Part model, mm, in its own coordinate system. A direction names the side the tool comes from. Coordinates: 2 decimals unless noted, no trailing zeros. Write each loop counter-clockwise with the first axis right and the second up, starting at its lowest first coordinate (ties: lowest second). Pieces come first, ordered by that corner, then holes. Notation, with made-up numbers: (14.25, 15) -> (73.25, 15) arc R18 ccw to (73.25, 25) -> close; hole circle Ø10 at (-8, 88). An arc over 180 degrees is marked (long way). Write item = value, one per line.
from build123d import *

# Parameters (mm, degrees)
SKETCH2_W           = 40
SKETCH2_H           = 30
BOSS_EXTRUDE1_DEPTH = 40
SKETCH3_W           = 10
SKETCH3_H           = 30
CUT_EXTRUDE1_DEPTH  = 40
CUT_EXTRUDE2_REACH  = 55.852
SKETCH5_R           = 2
FILLET2_R           = 1


with BuildPart() as part:
    # Sketch2 → Boss-Extrude1 (new body)
    with BuildSketch(Plane(origin=(0, 0, 0), x_dir=(1, 0, 0), z_dir=(0, 1, 0))):
        Rectangle(SKETCH2_W, SKETCH2_H)
    extrude(amount=BOSS_EXTRUDE1_DEPTH)

    # Sketch3 → Cut-Extrude1 (cut)
    with BuildSketch(Plane(origin=(20, 0, 0), x_dir=(0, 0, -1), z_dir=(1, 0, 0))):
        with Locations((5, 20)):
            Rectangle(SKETCH3_W, SKETCH3_H)
    extrude(amount=-CUT_EXTRUDE1_DEPTH, mode=Mode.SUBTRACT)

    # Sketch5 → Cut-Extrude2 (cut, up to next)
    with BuildSketch(Plane.XY.offset(15), mode=Mode.PRIVATE) as cut_extrude2_sk1:
        with Locations((12.5, 7.8)):
            Circle(SKETCH5_R)
    cut_extrude2_tool1 = extrude(cut_extrude2_sk1.sketch, amount=-CUT_EXTRUDE2_REACH, mode=Mode.PRIVATE) & part.part
    # Sketch5 → Cut-Extrude2 (cut, up to next)
    with BuildSketch(Plane.XY.offset(15), mode=Mode.PRIVATE) as cut_extrude2_sk2:
        with Locations((12.5, 32.8)):
            Circle(SKETCH5_R)
    cut_extrude2_tool2 = extrude(cut_extrude2_sk2.sketch, amount=-CUT_EXTRUDE2_REACH, mode=Mode.PRIVATE) & part.part
    # Sketch5 → Cut-Extrude2 (cut, up to next)
    with BuildSketch(Plane.XY.offset(15), mode=Mode.PRIVATE) as cut_extrude2_sk3:
        with Locations((-12.5, 32.8)):
            Circle(SKETCH5_R)
    cut_extrude2_tool3 = extrude(cut_extrude2_sk3.sketch, amount=-CUT_EXTRUDE2_REACH, mode=Mode.PRIVATE) & part.part
    # Sketch5 → Cut-Extrude2 (cut, up to next)
    with BuildSketch(Plane.XY.offset(15), mode=Mode.PRIVATE) as cut_extrude2_sk4:
        with Locations((-12.5, 7.8)):
            Circle(SKETCH5_R)
    cut_extrude2_tool4 = extrude(cut_extrude2_sk4.sketch, amount=-CUT_EXTRUDE2_REACH, mode=Mode.PRIVATE) & part.part
    add(cut_extrude2_tool1.solids().sort_by_distance((12.5, 7.8, 15))[0], mode=Mode.SUBTRACT)
    add(cut_extrude2_tool2.solids().sort_by_distance((12.5, 32.8, 15))[0], mode=Mode.SUBTRACT)
    add(cut_extrude2_tool3.solids().sort_by_distance((-12.5, 32.8, 15))[0], mode=Mode.SUBTRACT)
    add(cut_extrude2_tool4.solids().sort_by_distance((-12.5, 7.8, 15))[0], mode=Mode.SUBTRACT)

    # Fillet2
    fillet2_edges = [part.edges().sort_by_distance(p)[0] for p in [
        (20, 40, 0),
        (0, 40, -15),
        (-20, 40, 0),
        (0, 0, -15),
        (20, 0, 0),
        (0, 0, 15),
        (-20, 0, 0),
        (-20, 20, -15),
        (20, 20, -15),
        (20, 20, 15),
        (-20, 20, 15),
        (0, 40, 15),
    ]]
    fillet(fillet2_edges, radius=FILLET2_R)


solid = part.part
Q1. Pin check, flat tips, straight feed: pin 1 (3 mm diameter, centred on y = 7, z = -8, fed in from -X); pin 2 (2.5 mm diameter, centred on x = -12.5, y = 32.8, fed in from +Z). Stop position of each tip, or through.
Model answer:
pin_1 = through
pin_2 = -10
Q2. Mould opens along X. For faces 4 (the face through (12.24, 34.783, 7.605)), 5 (the face through (0, 35, -5)), 6 (the face through (-19.715, 20.266, 14.699)) say: released by +X, released by -X, zero draft, split by the parting line, or undercut.
Model answer:
face_4 = undercut
face_5 = zero draft
face_6 = released by -X
Q3. Probe line 1 (Y direction, x = 12.5, z = 4.75); line 2 (Z direction, x = 10, y = 17); line 3 (Y direction, x = -11, z = 2.5). List the from-to ranges inside material, lowest first. Write a range as from..to.
Model answer:
line_1 = 0..5.8, 9.8..30.8, 34.8..40
line_2 = -15..-10, 0..15
line_3 = 0..6.48, 9.12..31.48, 34.12..40
Q4. Which spindle directions (+Z, -Z, +X, -X, +Y, -Y) get a long thin tool onto all of the face, cutting with end or side? Do faces 1 (the face through (-20, 20, 3)), 2 (the face through (0, 20, -10)), 3 (the face through (-12.76, 34.783, 7.605)). Say none if no direction does.
Model answer:
face_1 = +Z, -Z, -X, +Y, -Y
face_2 = +X, -X
face_3 = +Z
Q5. Saw through at B-B on y = 7.8. Give the cut face in (x, z).
Model answer:
outline = (-20, -14) arc R1 ccw to (-19, -15) -> (19, -15) arc R1 ccw to (20, -14) -> (20, -10) -> (-20, -10) -> close; (-20, 0) -> (-14.5, 0) -> (-14.5, 15) -> (-19, 15) arc R1 ccw to (-20, 14) -> close; (-10.5, 0) -> (10.5, 0) -> (10.5, 15) -> (-10.5, 15) -> close; (14.5, 0) -> (20, 0) -> (20, 14) arc R1 ccw to (19, 15) -> (14.5, 15) -> close
Q6. Saw through at C-C on x = -12.5. Give the cut face in (y, z).
Model answer:
outline = (0, -14) arc R1 ccw to (1, -15) -> (39, -15) arc R1 ccw to (40, -14) -> (40, 14) arc R1 ccw to (39, 15) -> (34.8, 15) -> (34.8, 0) -> (35, 0) -> (35, -10) -> (5, -10) -> (5, 0) -> (5.8, 0) -> (5.8, 15) -> (1, 15) arc R1 ccw to (0, 14) -> close; (9.8, 0) -> (30.8, 0) -> (30.8, 15) -> (9.8, 15) -> close
Q7. Saw through at A-A on z = -7.5. Give the cut face in (x, y), and give its area (3 significant figures).
Model answer:
outline = (-20, 1) arc R1 ccw to (-19, 0) -> (19, 0) arc R1 ccw to (20, 1) -> (20, 5) -> (-20, 5) -> close; (-20, 35) -> (20, 35) -> (20, 39) arc R1 ccw to (19, 40) -> (-19, 40) arc R1 ccw to (-20, 39) -> close
area = 399 mm²
